Input: dimensioned drawing with shaded views. Units: mm. Origin: part minimum x, y, z. Round coordinates to 2 decimals unless told otherwise and drop trailing zeros. Write each loop counter-clockwise with the first axis right and the second up, starting at its lowest first coordinate (ties: lowest second). Pieces come first, ordered by that corner, then holes. Notation, with made-up numbers: M -19.75,10.25 L -15.75,10.25 A23 cw -15.75,23.25 Z; hole C -30,79.5 d9. An arc over 180 degrees is marked long. Put each result on its own line as item: value. Start each with the question number.
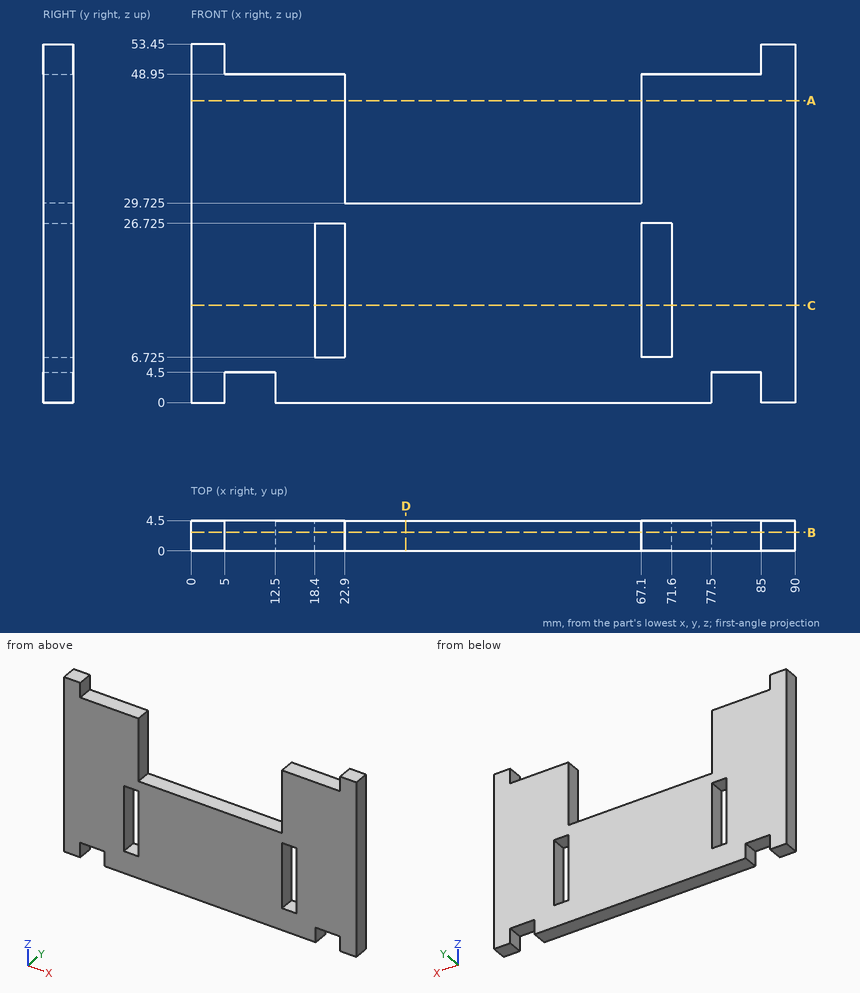
1) Section D-D, the plane x = 32. Output: boundary loops of the cut face in (y, z) (3 decimals), and give its area (3 significant figures).
2) Section A-A, the plane z = 45. Output: boundary loops of the cut face in (x, y).
3) Section B-B, the plane y = 2.75. Output: boundary loops of the cut face in (x, z) (3 decimals).
4) First-contact query: pin 1 (1.3 mm diameter, centred on x = 73, y = 1.5, fed in from +Z); pin 2 (2 mm diameter, centred on x = 34, y = 2, fed in from +Z) (3 decimals). Flat tips, straight axial feed; report the tip coordinate or a pass-through.
5) Section C-C, the plane z = 14.5. Output: boundary loops of the cut face in (x, y).
6) Ray query, probe 1 along X at (y, z) = (4.1, 26.5); probe 2 along X at (y, z) = (3.55, 33.5); probe 3 along Z at (x, y) = (69, 1.4) (3 decimals). Return the intervals inside material, ascending.
Solved:
1. outline: M 0,0 L 4.5,0 L 4.5,29.725 L 0,29.725 Z
1. area: 134 mm2
2. outline: M 0,0 L 22.9,0 L 22.9,4.5 L 0,4.5 Z; M 67.1,0 L 90,0 L 90,4.5 L 67.1,4.5 Z
3. outline: M 0,0 L 5,0 L 5,4.5 L 12.5,4.5 L 12.5,0 L 77.5,0 L 77.5,4.5 L 85,4.5 L 85,0 L 90,0 L 90,53.45 L 85,53.45 L 85,48.95 L 67.1,48.95 L 67.1,29.725 L 22.9,29.725 L 22.9,48.95 L 5,48.95 L 5,53.45 L 0,53.45 Z; hole M 18.4,6.725 L 22.9,6.725 L 22.9,26.725 L 18.4,26.725 Z; hole M 67.1,6.725 L 71.6,6.725 L 71.6,26.725 L 67.1,26.725 Z
4. pin 1: stops at z = 48.95
4. pin 2: stops at z = 29.725
5. outline: M 0,0 L 18.4,0 L 18.4,4.5 L 0,4.5 Z; M 22.9,0 L 67.1,0 L 67.1,4.5 L 22.9,4.5 Z; M 71.6,0 L 90,0 L 90,4.5 L 71.6,4.5 Z
6. probe 1: x = 0 to 18.4, 22.9 to 67.1, 71.6 to 90
6. probe 2: x = 0 to 22.9, 67.1 to 90
6. probe 3: z = 0 to 6.725, 26.725 to 48.95
